Input: part model. Units: mm. Frame: model coordinates. Face numbers are marked on the shaded views. A direction names the side the tool comes from. Round coordinates to 2 decimals unless told otherwise and drop trailing zeros. Loops run counter-clockwise (first coordinate to the right, second up) from the corner with the lowest first, then second, coordinate; pieces in that order, holes last. Notation, with made-up numbers: (16.25, -3) -> (57.25, -3) arc R17 ccw to (57.25, 8) -> close; hole circle Ø4 at (-21.5, 31). An arc over 180 degrees is marked (long way). Answer as a JSON object with one key per item and string values.
```python
from build123d import *

# Parameters (mm, degrees)
EXTRUDE_1_DEPTH             = 10
FILLET_1_R                  = 2
HOLE_WIZARD_M31_D           = 3.4
HOLE_WIZARD_M31_DEPTH       = 6
HOLE_WIZARD_M31_CBORE_D     = 6.5
HOLE_WIZARD_M31_CBORE_DEPTH = 3
M3X0_51_D                   = 2.5
M3X0_51_DEPTH               = 6
M3X0_52_D                   = 2.5


with BuildPart() as part:
    # Эскиз1 → Бобышка-Вытянуть1 (new body)
    with BuildSketch(Plane.XY):
        with BuildLine():
            Line((-14, 0), (-14, -64))
            Line((-14, -64), (-8, -64))
            Line((-8, -64), (-8, -7.549834435))
            ThreePointArc((-8, -7.549834435), (6.149683661, 9.120383264), (-4, -10.246950766))
            Line((-4, -10.246950766), (-4, -24))
            Line((-4, -24), (2, -24))
            Line((2, -24), (2, -13.856406461))
            ThreePointArc((2, -13.856406461), (9.16515139, 10.583005244), (-14, 0))
        make_face()
    extrude(amount=EXTRUDE_1_DEPTH)

    # Скругление1
    fillet_1_edges = [part.edges().sort_by_distance(p)[0] for p in [
        (2, -13.856406461, 5),
        (2, -24, 5),
        (-4, -24, 5),
        (-4, -10.246950766, 5),
        (-8, -7.549834435, 5),
        (-8, -64, 5),
        (-14, -64, 5),
    ]]
    fillet(fillet_1_edges, radius=FILLET_1_R)

    # Цековка для винта с внутренним шестигранником M31
    with Locations(Plane.ZY.offset(14)):
        with Locations((5, -18.745966692)):
            CounterBoreHole(HOLE_WIZARD_M31_D / 2, HOLE_WIZARD_M31_CBORE_D / 2, HOLE_WIZARD_M31_CBORE_DEPTH, depth=HOLE_WIZARD_M31_DEPTH)

    # Отверстие обработанное метчиком M3x0.51
    with Locations(Plane.ZY.offset(4)):
        with Locations((5, -18.745966692)):
            Hole(M3X0_51_D / 2, depth=M3X0_51_DEPTH)

    # Отверстие обработанное метчиком M3x0.52 (through all)
    with Locations(Plane.ZY.offset(14)):
        with Locations((5, -27), (5, -59)):
            Hole(M3X0_52_D / 2)


solid = part.part
```
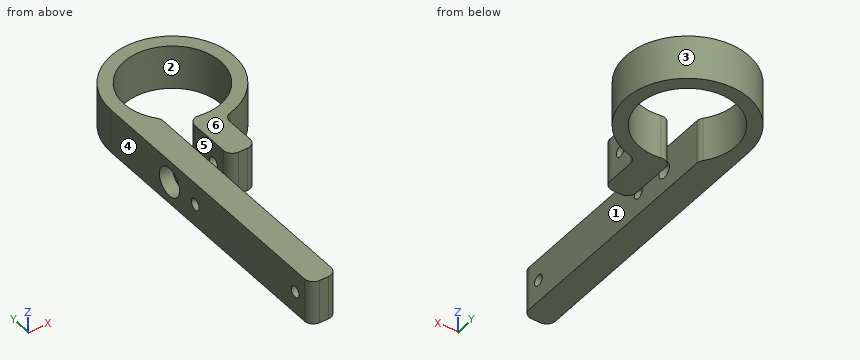
1) Section B-B, the plane x = 1. Output: boundary loops of the cut face in (y, z).
Output:
{"outline": "(-23.73, 0) -> (-10.95, 0) -> (-10.95, 10) -> (-23.73, 10) -> close; (10.95, 0) -> (13.96, 0) -> (13.96, 10) -> (10.95, 10) -> close; hole circle Ø2.5 at (-18.75, 5)"}
2) Draft query along X for the marked faces 1, 2, 3 and 4. Return one class per face: +X half, -X half, draft (parallel to the pull), parting line (faces both ways), or undercut.
Output:
{"face 1": "undercut", "face 2": "undercut", "face 3": "parting line", "face 4": "-X half"}
3) Section D-D, the plane z = 5.25. Count the separate pieces of the cut face and the enclosed holes in it, plus the area to 3 significant figures.
Output:
{"separate pieces": "5", "enclosed holes": "0", "area": "540 mm^2"}
4) Section C-C, the plane x = 6.5. Output: boundary loops of the cut face in (y, z).
Output:
{"outline": "(-12.4, 0) -> (-8.87, 0) -> (-8.87, 10) -> (-12.4, 10) -> close; (8.87, 0) -> (12.4, 0) -> (12.4, 10) -> (8.87, 10) -> close"}
5) Ray query, probe 1 along Y at (x, z) = (0.1, 5); probe 2 along X at (y, z) = (0, 5); probe 3 along Y at (x, z) = (-11.65, 5). Return the intervals inside material, ascending.
Output:
{"probe 1": "y = -24 to -20, -17.5 to -11, 11 to 14", "probe 2": "x = -14 to -11, 11 to 14", "probe 3": "y = -64 to -60.25, -57.75 to -28.25, -25.75 to -22, -15.5 to 7.76"}
6) Section A-A, the plane y = -59. Output: boundary loops of the cut face in (x, z), plus the area to 3 significant figures.
Output:
{"outline": "(-14, 0) -> (-8, 0) -> (-8, 3.75) -> (-14, 3.75) -> close; (-14, 6.25) -> (-8, 6.25) -> (-8, 10) -> (-14, 10) -> close", "area": "45.0 mm^2"}
7) Reachability of the marked faces 5 and 6 from +Z, -Z, +X, -X, +Y, -Y: full face, straight path, thin tool, end or side. Return the list, or none.
Output:
{"face 5": "+Z, -Z, -Y", "face 6": "+Z, +X, -X, +Y, -Y"}
8) Contact query for flat-ended pins moving along their axis: P1, Ø3, axis at y = -27, z = 5, coming from the +X side; P2, Ø3, axis at y = -18.75, z = 5, coming from the -X side; P3, Ø2, axis at x = -11, z = 7.5, coming from the +Y side. Output: stop coordinate, or through.
Output:
{"P1": "stops at x = -8", "P2": "stops at x = -4", "P3": "stops at y = 9.8"}
